from build123d import *

# Parameters (mm, degrees)
F0_R     = 2.95
F1_DEPTH = 9
F0_R_2   = 5
F0_R_3   = 3.125
F2_DEPTH = 1
F3_DEPTH = 12
F4_R     = 1


with BuildPart() as f1:
    # F0 (on Top) → F1 (new body)
    with BuildSketch(Plane.XY):
        Circle(F0_R)
    extrude(amount=F1_DEPTH)

    # F0 (on Top) → F2 (join)
    with BuildSketch(Plane.XY):
        Circle(F0_R_2)
        Circle(F0_R_3, mode=Mode.SUBTRACT)
        Circle(F0_R_3)
        Circle(F0_R, mode=Mode.SUBTRACT)
    extrude(amount=F2_DEPTH)

    # F0 (on Top) → F3 (join)
    with BuildSketch(Plane.XY):
        Circle(F0_R_3)
        Circle(F0_R, mode=Mode.SUBTRACT)
        Circle(F0_R)
    extrude(amount=-F3_DEPTH)

    # F4
    f4_edges = [f1.edges().sort_by_distance(p)[0] for p in [
        (-3.125, 0, -12),
    ]]
    fillet(f4_edges, radius=F4_R)


solid = f1.part
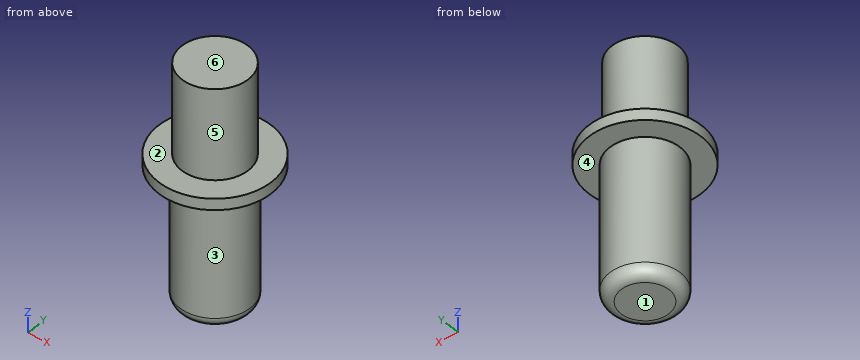
Read the model definition and answer for the solid it produces. Units are mm, in the model's axes. Face numbers are marked on the shaded views. A direction names the side the tool comes from. Give positions to 0.01 mm unless a question says otherwise; leave off trailing zeros. Loops run counter-clockwise (first coordinate to the right, second up) from the corner with the lowest first, then second, coordinate; pieces in that order, holes last. Notation, with made-up numbers: (-11, 29) - (-7, 29) arc R8 ccw to (-7, 39) - close; hole circle Ø2 at (69, 7.5). An arc over 180 degrees is marked (long way). Answer as CSV lines item,"result". Start each with the question number.
1) Which of the six approach directions +Z, -Z, +X, -X, +Y, -Y give full straight-line access (tool end or side, diameter ignored) to the marked faces 4, 5 and 6?
2) Find section C-C (z = -6.5). Write down the section's boundary in (x, y) (3 decimals), then the cut area to 3 significant figures.
3) Find section D-D (z = 7.75). Write down the section's boundary in (x, y).
4) Each of these flat-tipped pins is pushed along its axis until it touches: pin 1 Ø1.5 at (x, y) = (-4, 0) entering from +Z; pin 2 Ø4 at (x, z) = (1.5, 2.5) entering from -Y; pin 3 Ø2 at (x, z) = (-4, 0.5) entering from -Y. Where does it stop, or does it pass through?
5) Find section A-A (x = 0). Write down the section's boundary in (y, z) (3 decimals).
6) Straight lines are drawn through the part: L1, parallel to Z at x = -3.75, y = 2.75; L2, parallel to Y at x = 0, z = -8.75 (3 decimals); L3, parallel to Y at x = -2, z = 4.75. For each, find the intervals that lie inside material, in ascending order. Write a range as from..to.
7) Determine the mould class of the marked faces 1, 2 and 3 for opening direction Z: released by +Z, released by -Z, zero draft, split by the parting line, or undercut.
Findings below:
1,face 4,"-Z"
1,face 5,"+Z"
1,face 6,"+Z, +X, -X, +Y, -Y"
2,outline,"circle Ø6.25 at (0, 0)"
2,area,"30.7 mm^2"
3,outline,"circle Ø5.9 at (0, 0)"
4,pin 1,"z = 1"
4,pin 2,"y = -5"
4,pin 3,"y = -4"
5,outline,"(-5, 0) - (-3.125, 0) - (-3.125, -11) arc R1 ccw to (-2.125, -12) - (2.125, -12) arc R1 ccw to (3.125, -11) - (3.125, 0) - (5, 0) - (5, 1) - (2.95, 1) - (2.95, 9) - (-2.95, 9) - (-2.95, 1) - (-5, 1) - close"
6,L1,"0..1"
6,L2,"-3.125..3.125"
6,L3,"-2.17..2.17"
7,face 1,"released by -Z"
7,face 2,"released by +Z"
7,face 3,"zero draft"
